```python
from build123d import *

# Parameters (mm, degrees)
BOX_W           = 100
BOX_H           = 6
BOX_DEPTH       = 76.7
SKETCH_W        = 60
SKETCH_H        = 95
PAD_DEPTH       = 96.4
SKETCH001_W     = 90
SKETCH001_H     = 90
POCKET_DEPTH    = 86.4
SKETCH003_R     = 11.5
SKETCH003_R_2   = 3.1
POCKET001_DEPTH = 20
SKETCH004_R     = 4.2
POCKET002_DEPTH = 13


with BuildPart() as crossbeam_slot:
    # Box → Box (new body)
    with BuildSketch(Plane(origin=(-100, 0, 10), x_dir=(1, 0, 0), z_dir=(0, 0, 1))):
        with Locations((50, 3)):
            Rectangle(BOX_W, BOX_H)
    extrude(amount=BOX_DEPTH)


with BuildPart() as pocket002:
    # Sketch → Pad (new body)
    with BuildSketch(Plane.XY):
        with Locations((-20, -41.5)):
            Rectangle(SKETCH_W, SKETCH_H)
    extrude(amount=PAD_DEPTH)

    # Cut: cut Crossbeam Slot
    add(crossbeam_slot.part, mode=Mode.SUBTRACT)

    # Sketch001 → Pocket (cut)
    with BuildSketch(Plane.XY.offset(96.4)):
        with Locations((-48, -58)):
            Rectangle(SKETCH001_W, SKETCH001_H)
    extrude(amount=-POCKET_DEPTH, mode=Mode.SUBTRACT)

    # Sketch003 → Pocket001 (cut)
    with BuildSketch(Plane.YZ.offset(10)):
        with Locations((-54.5, 65)):
            Circle(SKETCH003_R)
        with Locations((-42, 43.349365)):
            Circle(SKETCH003_R_2)
        with Locations((-42, 86.650635)):
            Circle(SKETCH003_R_2)
        with Locations((-79.5, 65)):
            Circle(SKETCH003_R_2)
    extrude(amount=-POCKET001_DEPTH, mode=Mode.SUBTRACT)

    # Sketch004 → Pocket002 (cut)
    with BuildSketch(Plane(origin=(0, 0, 0), x_dir=(-1, 0, 0), z_dir=(0, 1, 0))):
        with Locations((8, 76.4)):
            Circle(SKETCH004_R)
        with Locations((40, 76.4)):
            Circle(SKETCH004_R)
        with Locations((8, 20)):
            Circle(SKETCH004_R)
        with Locations((40, 20)):
            Circle(SKETCH004_R)
    extrude(amount=-POCKET002_DEPTH, mode=Mode.SUBTRACT)


solid = pocket002.part
```
Could you check a few things on this model? Use its own coordinates, in mm. A direction names the side the tool comes from. Give positions to 0.01 mm unless a question says otherwise; leave off trailing zeros. Loops run counter-clockwise (first coordinate to the right, second up) from the corner with the lowest first, then second, coordinate; pieces in that order, holes last. Notation, with made-up numbers: (65, 74.25) - (109, 74.25) arc R11 cw to (109, 83.25) - close; hole circle Ø11 at (89, -38). An arc over 180 degrees is marked (long way). Use one line per item in the form item = value.
1. I need wall thicknesses on probe 1 along Z at (x, y) = (-40, -6); probe 2 along Z at (x, y) = (-13.5, -47.5); probe 3 along X at (y, z) = (-7.5, 23). Which ranges of each line are inside material? Lowest first, please.
Response values:
probe_1 = 0 to 15.8, 24.2 to 72.2, 80.6 to 96.4
probe_2 = 0 to 10
probe_3 = -50 to -42.94, -37.06 to -10.94, -5.06 to 10
2. I'm going to push flat-ended pins straight in: pin 1 Ø1 at (y, z) = (-65, 15) entering from -X; pin 2 Ø9.5 at (x, z) = (-8, 20) entering from +Y; pin 3 Ø8 at (x, z) = (-15, 85.5) entering from -Y; pin 4 Ø5 at (y, z) = (1.5, 41) entering from -X. Where does each tip first touch, or does it pass through?
Response values:
pin_1 = -3
pin_2 = 0
pin_3 = -13
pin_4 = -50
3. I want a section at C-C (z = 33.5). Please give me the cut outline in (x, y), and give its area (3 significant figures).
Response values:
outline = (-50, -13) - (-3, -13) - (-3, -89) - (10, -89) - (10, 6) - (0, 6) - (0, 0) - (-50, 0) - close
area = 1,830 mm²
4. I want a section at D-D (x = -32.5). Please give me the cut outline in (y, z), and give its area (3 significant figures).
Response values:
outline = (-89, 0) - (6, 0) - (6, 10) - (0, 10) - (0, 86.7) - (6, 86.7) - (6, 96.4) - (-13, 96.4) - (-13, 10) - (-89, 10) - close
area = 2,130 mm²
5. Thinking about a two-plate mould opening in Y: for faces 1 (the face through (3.59, -40.57, 83.9)), 2 (the face through (-27, -13, 54)), 3 (the face through (0, 3, 48)), which applies, released by +Y, released by -Y, zero draft, split by the parting line, or undercut?
Response values:
face_1 = undercut
face_2 = released by -Y
face_3 = zero draft
6. On a 3-axis mill with a long thin cutter (end or side, diameter ignored), from which of +Z, -Z, +X, -X, +Y, -Y can I reach the whole of each face in a straight line? I mean faces 4 (the face through (3.591, -39.136, 42.162)), 5 (the face through (-27, -50, 10)), 6 (the face through (-25, 3, 86.7)). Say none if no direction works.
Response values:
face_4 = +X, -X
face_5 = +Z, -X, -Y
face_6 = -X, +Y
7. I want a section at B-B (y = -79.5). Please give me the cut outline in (x, z), and give its area (3 significant figures).
Response values:
outline = (-50, 0) - (10, 0) - (10, 61.9) - (-3, 61.9) - (-3, 10) - (-50, 10) - close; (-3, 68.1) - (10, 68.1) - (10, 96.4) - (-3, 96.4) - close
area = 1,640 mm²
8. I want a section at A-A (x = -8). Please give me the cut outline in (y, z), and give its area (3 significant figures).
Response values:
outline = (-89, 0) - (6, 0) - (6, 10) - (0, 10) - (0, 15.8) - (-13, 15.8) - (-13, 10) - (-89, 10) - close; (-13, 24.2) - (0, 24.2) - (0, 72.2) - (-13, 72.2) - close; (-13, 80.6) - (0, 80.6) - (0, 86.7) - (6, 86.7) - (6, 96.4) - (-13, 96.4) - close
area = 1,910 mm²
